Model file for the job. Use its own axes, mm. A direction names the side the tool comes from. Give positions to 0.01 mm unless a question says otherwise; leave off trailing zeros. Loops run counter-clockwise (first coordinate to the right, second up) from the corner with the lowest first, then second, coordinate; pieces in that order, holes last. Notation, with made-up numbers: M 12.25,-11 L 41.25,-11 A25 ccw 41.25,13 Z; hole C -10.75,-25.75 d5. An arc over 180 degrees is marked long. Answer in a Markdown table with one row per item.
```python
from build123d import *

# Parameters (mm, degrees)
F0_W     = 98
F0_H     = 57
F1_DEPTH = 21
F2_W     = 5
F2_H     = 8
F3_DEPTH = 15
F4_W     = 12
F4_H     = 11
F5_DEPTH = 5


with BuildPart() as f1:
    # F0 (on Top) → F1 (new body)
    with BuildSketch(Plane.XY):
        with Locations((49, 28.5)):
            Rectangle(F0_W, F0_H)
    extrude(amount=F1_DEPTH)

    # F2 (on face) → F3 (join)
    with BuildSketch(Plane(origin=(0, 57, 0), x_dir=(-1, 0, 0), z_dir=(0, 1, 0))):
        with Locations((-95.5, 10.5)):
            Rectangle(F2_W, F2_H)
    extrude(amount=F3_DEPTH)

    # F4 (on face) → F5 (join)
    with BuildSketch(Plane.XZ):
        with Locations((92, 10.5)):
            Rectangle(F4_W, F4_H)
    extrude(amount=F5_DEPTH)


solid = f1.part
```
Q1. Drop flat-ended pins along their axis: pin 1 (5 mm diameter, centred on x = 72, z = 8.5, fed in from -Y); pin 2 (5.5 mm diameter, centred on x = 95, y = 63.5, fed in from -Z); pin 3 (4 mm diameter, centred on y = -3.5, z = 13, fed in from -X). Give the stop position or say it passes through.
Reported:
| item | result |
|---|---|
| pin 1 | y = 0 |
| pin 2 | z = 6.5 |
| pin 3 | x = 86 |
Q2. Probe probe 1 along Y at (x, z) = (40, 13.5); probe 2 along Y at (x, z) = (92.5, 13.5). List the from-to ranges inside material, lowest first.
Reported:
| item | result |
|---|---|
| probe 1 | 0 to 57 |
| probe 2 | -5 to 57 |
Q3. 3-axis set-ups, long thin cutter, end or side, ignore diameter. For faces 1 (the face through (92, -2, 16)), 2 (the face through (93, 64, 10)), 3 (the face through (86, -2, 10)): which of +Z, -Z, +X, -X, +Y, -Y reach the whole face in a straight line?
Reported:
| item | result |
|---|---|
| face 1 | +Z, +X, -X, -Y |
| face 2 | +Z, -Z, -X, +Y |
| face 3 | +Z, -Z, -X, -Y |
Q4. Saw through at B-B (x = 21). Give the cut face in (y, z).
Reported:
| item | result |
|---|---|
| outline | M 0,0 L 57,0 L 57,21 L 0,21 Z |
Q5. Saw through at C-C (y = 61). Give the cut face in (x, z), and give its area (3 significant figures).
Reported:
| item | result |
|---|---|
| outline | M 93,6.5 L 98,6.5 L 98,14.5 L 93,14.5 Z |
| area | 40.0 mm² |
Q6. Saw through at A-A (z = 12.25). Give the cut face in (x, y), and give its area (3 significant figures).
Reported:
| item | result |
|---|---|
| outline | M 0,0 L 86,0 L 86,-5 L 98,-5 L 98,72 L 93,72 L 93,57 L 0,57 Z |
| area | 5,720 mm² |
